from build123d import *

# Parameters (mm, degrees)
SKETCH_W      = 203.2
SKETCH_H      = 44.45
SKETCH_R      = 2.775
SKETCH_W_2    = 159
SKETCH_H_2    = 26
PAD_DEPTH     = 2.2
SKETCH001_W   = 163
SKETCH001_H   = 30
SKETCH001_W_2 = 159
SKETCH001_H_2 = 26
PAD001_DEPTH  = 98.8
SKETCH002_W   = 163
SKETCH002_H   = 30
SKETCH002_W_2 = 143
SKETCH002_H_2 = 26
PAD002_DEPTH  = 2


with BuildPart() as part:
    # Sketch → Pad (new body)
    with BuildSketch(Plane.XY):
        Rectangle(SKETCH_W, SKETCH_H)
        with Locations((-93.6625, 15.875)):
            Circle(SKETCH_R, mode=Mode.SUBTRACT)
        with Locations((-93.6625, -15.875)):
            Circle(SKETCH_R, mode=Mode.SUBTRACT)
        with Locations((93.6625, 15.875)):
            Circle(SKETCH_R, mode=Mode.SUBTRACT)
        with Locations((93.6625, -15.875)):
            Circle(SKETCH_R, mode=Mode.SUBTRACT)
        Rectangle(SKETCH_W_2, SKETCH_H_2, mode=Mode.SUBTRACT)
    extrude(amount=PAD_DEPTH)

    # Sketch001 (on Face14 of Pad) → Pad001 (join)
    with BuildSketch(Plane.XY.offset(2.2)):
        Rectangle(SKETCH001_W, SKETCH001_H)
        Rectangle(SKETCH001_W_2, SKETCH001_H_2, mode=Mode.SUBTRACT)
    extrude(amount=PAD001_DEPTH)

    # Sketch002 (on Face15 of Pad001) → Pad002 (join)
    with BuildSketch(Plane.XY.offset(101)):
        Rectangle(SKETCH002_W, SKETCH002_H)
        Rectangle(SKETCH002_W_2, SKETCH002_H_2, mode=Mode.SUBTRACT)
    extrude(amount=PAD002_DEPTH)


solid = part.part
CAD build for the part. Positions are in the model's coordinates, mm. A direction names the side the tool comes from. Round coordinates to 2 decimals unless told otherwise and drop trailing zeros. Write each loop counter-clockwise with the first axis right and the second up, starting at its lowest first coordinate (ties: lowest second). Pieces come first, ordered by that corner, then holes. Notation, with made-up numbers: M -36,27.25 L -30,27.25 A21 cw -30,35.25 Z; hole C 88.25,56 d1. An arc over 180 degrees is marked long. Use a Markdown table: item, result. Add a question column.
1. Slice it at B-B on x = 32. Give the cut face in (y, z) (3 decimals), then the cut area to 3 significant figures.
2. 3-axis set-ups, long thin cutter, end or side, ignore diameter. For faces 4 (the face through (-1, -15, 52)), 5 (the face through (81.5, 0, 52)), 6 (the face through (75, 0, 101)), 7 (the face through (-91.1, 14.81, 1.08)), 8 (the face through (-1, -15, 0)): which of +Z, -Z, +X, -X, +Y, -Y reach the whole face in a straight line?
3. Slice it at D-D on x = 74. Give the cut face in (y, z) (3 decimals), then the cut area to 3 significant figures.
4. Pull direction Y, two halves, no side cores. Call faces 1 (the face through (-81.5, 0, 52)), 2 (the face through (-1, 15, 52)), 3 (the face through (79.5, 0, 50)): released by +Y, released by -Y, zero draft, split by the parting line, or undercut.
5. Slice it at C-C on z = 65. Give the cut face in (x, y), then the cut area to 3 significant figures.
6. Flat gauge pins, fed straight in: P1, Ø6.5, axis at x = -74, y = 2, coming from the -Z side; P2, Ø5, axis at y = 0, z = 11, coming from the -X side; P3, Ø8, axis at y = -15.5, z = 31.5, coming from the +X side; P4, Ø4, axis at x = 14, y = -10, coming from the -Z side. Where does each tip first touch, or does it go through?
7. Drill centre lines: probe 1 along Y at (x, z) = (-20, 59); probe 2 along X at (y, z) = (2.5, 83.5); probe 3 along Z at (x, y) = (-91, -9). Where is each one in solid material? Low to high.
8. Slice it at A-A on y = 9. Give the cut face in (x, z), then the cut area to 3 significant figures.
Reply:
| question | item | result |
|---|---|---|
| 1 | outline | M -22.225,0 L -13,0 L -13,103 L -15,103 L -15,2.2 L -22.225,2.2 Z; M 13,0 L 22.225,0 L 22.225,2.2 L 15,2.2 L 15,103 L 13,103 Z |
| 1 | area | 444 mm^2 |
| 2 | face 4 | +Z, +X, -X, -Y |
| 2 | face 5 | +Z, +X, +Y, -Y |
| 2 | face 6 | -Z |
| 2 | face 7 | +Z, -Z |
| 2 | face 8 | -Z, +X, -X, +Y, -Y |
| 3 | outline | M -22.225,0 L -13,0 L -13,101 L 13,101 L 13,0 L 22.225,0 L 22.225,2.2 L 15,2.2 L 15,103 L -15,103 L -15,2.2 L -22.225,2.2 Z |
| 3 | area | 496 mm^2 |
| 4 | face 1 | zero draft |
| 4 | face 2 | released by +Y |
| 4 | face 3 | undercut |
| 5 | outline | M -81.5,-15 L 81.5,-15 L 81.5,15 L -81.5,15 Z; hole M -79.5,-13 L 79.5,-13 L 79.5,13 L -79.5,13 Z |
| 5 | area | 756 mm^2 |
| 6 | P1 | stops at z = 101 |
| 6 | P2 | stops at x = -81.5 |
| 6 | P3 | stops at x = 81.5 |
| 6 | P4 | passes through |
| 7 | probe 1 | y = -15 to -13, 13 to 15 |
| 7 | probe 2 | x = -81.5 to -79.5, 79.5 to 81.5 |
| 7 | probe 3 | z = 0 to 2.2 |
| 8 | outline | M -101.6,0 L -79.5,0 L -79.5,101 L -71.5,101 L -71.5,103 L -81.5,103 L -81.5,2.2 L -101.6,2.2 Z; M 71.5,101 L 79.5,101 L 79.5,0 L 101.6,0 L 101.6,2.2 L 81.5,2.2 L 81.5,103 L 71.5,103 Z |
| 8 | area | 532 mm^2 |
